Geometry check sheet. Reference: drawing and pictorial views, mm from the part's lowest x, y, z. A direction names the side the tool comes from. Coordinates: 2 decimals unless noted, no trailing zeros. Loops run counter-clockwise (first coordinate to the right, second up) from the corner with the lowest first, then second, coordinate; pieces in that order, holes last. Notation, with made-up numbers: (52.5, -30) - (87.5, -30) arc R17 cw to (87.5, -4) - close; hole circle Ø4 at (-3.75, 10.5). An arc over 180 degrees is marked (long way). Write each question's results on one line, items separated by ' | '. Start each with the question number.
1. Tool access check on the marked faces 1 and 2. Record the directions out of +Z, -Z, +X, -X, +Y, -Y that give a thin tool (end or side, any length) a straight path to the whole face; none if there is none.
2. Cross-section at D-D (z = 9.5). Record the cut outline in (x, y).
3. Cross-section at B-B (x = 12.25). Record the cut outline in (y, z) (3 decimals), and give its area (3 significant figures).
4. Gauge pin test, flat ends, axial feed: P1, Ø12, axis at x = 16.5, z = 9, coming from the +Y side; P2, Ø12, axis at x = 20.5, y = 55.5, coming from the +Z side; P3, Ø3, axis at x = 16, y = 17, coming from the +Z side; P4, Ø6, axis at x = 15.5, y = 7, coming from the +Z side. Record the tip position at first contact, or that the pin passes through.
5. Thickness scan on line 1 (Y direction, x = 22.25, z = 17.75); line 2 (Y direction, x = 15.5, z = 11.5); line 3 (Z direction, x = 12, y = 9.5). Record the ranges inside material, lowest first. Write a range as [from, to].
6. Cross-section at C-C (y = 44). Record the cut outline in (x, z) (3 decimals).
7. Cross-section at A-A (z = 12.25). Record the cut outline in (x, y) (3 decimals).
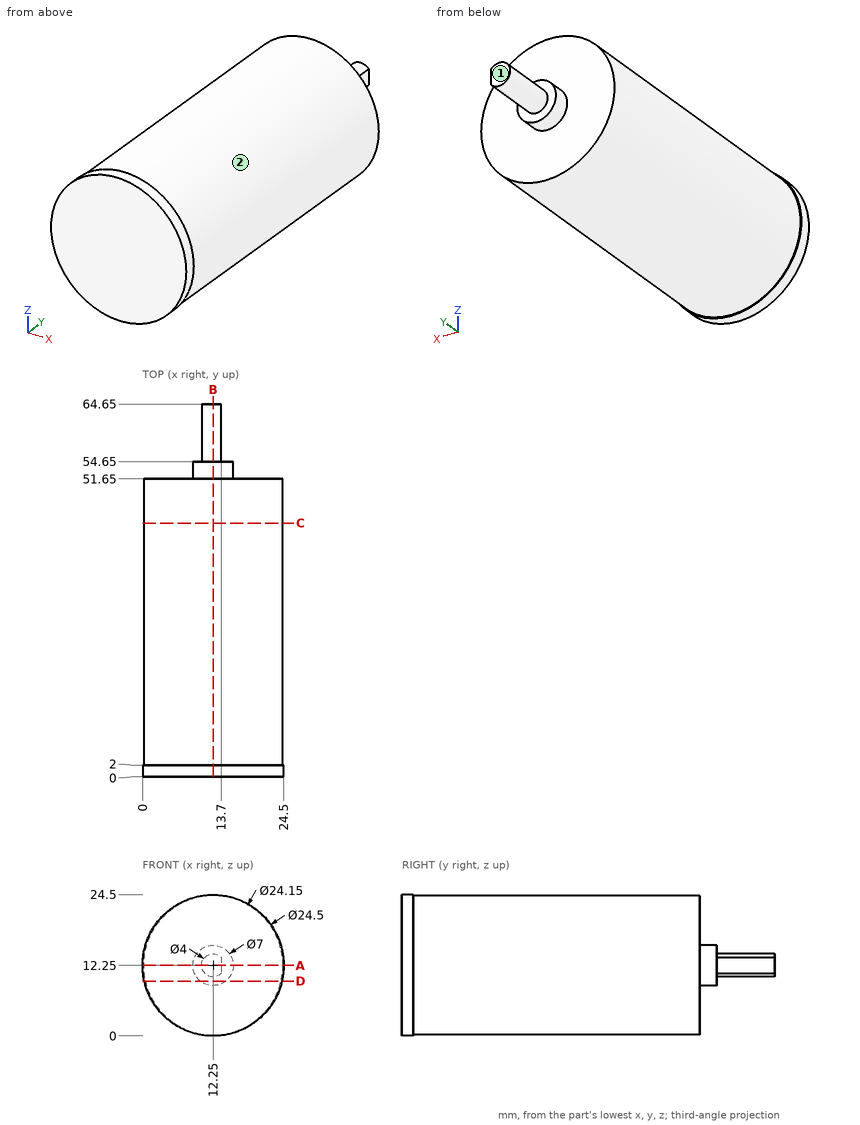
Established:
1) face 1: +Z, -Z, +X, -X, +Y | face 2: +Y
2) outline: (0.31, 0) - (24.19, 0) - (24.19, 2) - (24.01, 2) - (24.01, 51.65) - (14.42, 51.65) - (14.42, 54.65) - (10.08, 54.65) - (10.08, 51.65) - (0.49, 51.65) - (0.49, 2) - (0.31, 2) - close
3) outline: (0, 0) - (2, 0) - (2, 0.175) - (51.65, 0.175) - (51.65, 8.75) - (54.65, 8.75) - (54.65, 10.25) - (64.65, 10.25) - (64.65, 14.25) - (54.65, 14.25) - (54.65, 15.75) - (51.65, 15.75) - (51.65, 24.325) - (2, 24.325) - (2, 24.5) - (0, 24.5) - close | area: 1,310 mm^2
4) P1: y = 64.65 | P2: z = 23.76 | P3: z = 24.11 | P4: z = 24.32
5) line 1: [0, 51.65] | line 2: [0, 54.65] | line 3: [0.18, 24.32]
6) outline: circle Ø24.15 at (12.25, 12.25)
7) outline: (0, 0) - (24.5, 0) - (24.5, 2) - (24.325, 2) - (24.325, 51.65) - (15.75, 51.65) - (15.75, 54.65) - (13.7, 54.65) - (13.7, 64.65) - (10.25, 64.65) - (10.25, 54.65) - (8.75, 54.65) - (8.75, 51.65) - (0.175, 51.65) - (0.175, 2) - (0, 2) - close
